Check sheet for the modelled part. Datum: model origin and axes. Units: mm. Face numbers are marked on the shaded views. A direction names the side the tool comes from. Round coordinates to 2 decimals unless told otherwise and drop trailing zeros. Write each loop counter-clockwise with the first axis right and the second up, starting at its lowest first coordinate (ties: lowest second). Pieces come first, ordered by that corner, then holes. Notation, with made-up numbers: (65, 72) - (109, 72) arc R14 ccw to (109, 81) - close; hole circle Ø6 at (76.25, 16.25). An arc over 180 degrees is marked (long way). Use one line per item in the form item = value. Start each with the question number.
1) Section check A-A (z = -2). Record the boundary of the cut face in (x, y) (3 decimals), then the cut area to 3 significant figures.
2) Scan lines: probe 1 along Z at (x, y) = (1.75, -2.75); probe 2 along Y at (x, z) = (0.75, -3); probe 3 along Y at (x, z) = (-1.75, -16). Record each from-to range of solid material in increasing order.
3) Set-up check for the marked faces 1 and 2: record each of +Z, -Z, +X, -X, +Y, -Y from which the full face is reachable in a straight line by a thin tool's end or side.
4) Gauge pin test, flat ends, axial feed: P1, Ø6, axis at x = 4, z = -18, coming from the -Y side; P2, Ø5, axis at y = 0.5, z = -9.5, coming from the +X side (3 decimals); P3, Ø3, axis at x = 0, z = -16.5, coming from the -Y side (3 decimals). Record the tip position at first contact, or that the pin passes through.
5) Draft check along X on the marked faces 3, 4 and 5. Enter one of: +X half, -X half, draft (parallel to the pull), parting line (faces both ways), or undercut.
from build123d import *

# Parameters (mm, degrees)
SKETCH001_R  = 7.415805
POCKET_DEPTH = 30.1762
CHAMFER_SIZE = 1


with BuildPart() as part:
    # Sketch → Revolution (revolve)
    with BuildSketch(Plane.XZ):
        Polygon((0, 4.7752), (5.55625, 4.7752), (6.4158, 4.374385), (6.4158, 0), (3.175, 0), (3.175, -25.4), (0, -25.4), align=None)
    revolve(axis=Axis((0, 0, 0), (0, 0, 1)))

    # Sketch001 → Pocket (cut, through all)
    with BuildSketch(Plane(origin=(0, 0, 4.7752), x_dir=(-1, 0, 0), z_dir=(0, 0, 1))):
        Circle(SKETCH001_R)
        Polygon((-3.207902, 5.55625), (3.207902, 5.55625), (6.415805, 0), (3.207902, -5.55625), (-3.207902, -5.55625), (-6.415805, 0), align=None, mode=Mode.SUBTRACT)
    extrude(amount=-POCKET_DEPTH, mode=Mode.SUBTRACT)

    # Chamfer
    chamfer_edges = [part.edges().sort_by_distance(p)[0] for p in [
        (-3.175, 0, -25.4),
    ]]
    chamfer(chamfer_edges, length=CHAMFER_SIZE)


solid = part.part
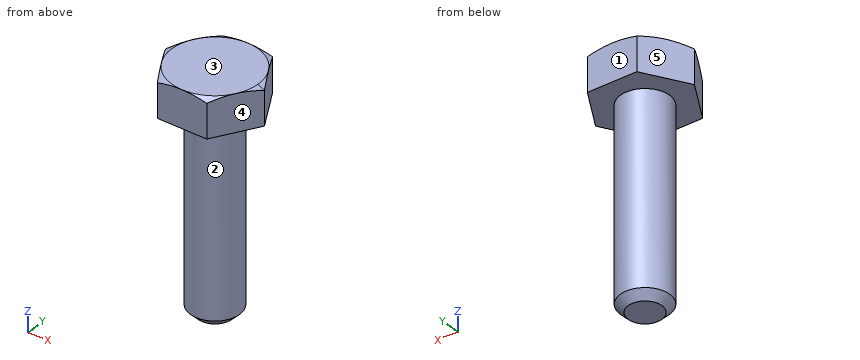
Results are:
q1.outline = circle Ø6.35 at (0, 0)
q1.area = 31.7 mm²
q2.probe_1 = 0 to 4.78
q2.probe_2 = -3.09 to 3.09
q2.probe_3 = -2.65 to 2.65
q3.face_1 = +Z, -Z, +X, -X, +Y
q3.face_2 = -Z
q4.P1 = -3.01
q4.P2 = 3.175
q4.P3 = -3.175
q5.face_3 = draft
q5.face_4 = +X half
q5.face_5 = -X half
